The listing builds one solid part. Answer for the finished solid, in the listing's coordinates (mm). Give positions to 0.01 mm unless a question says otherwise; leave off trailing zeros. Order: outer loops, then holes, each group sorted by start corner. A loop starts at its lowest first (then second) coordinate and runs counter-clockwise, first axis right, second up. Notation, with made-up numbers: (45.25, 87.25) - (64.25, 87.25) arc R18 cw to (64.25, 116.25) - close; hole circle Ø11 at (-22, 28.5). An arc over 180 degrees is marked (long way). Answer as a JSON object with one key per item and string values. Group by question number.
Q1. The mould has two halves that part along X. Classify faces 1 (the face through (-7.535, 4.27, 0.068)), 2 (the face through (7.535, -4.27, 0.068)), 3 (the face through (-2.285, 3.584, 0.059)): released by +X, released by -X, zero draft, split by the parting line, or undercut.
Q2. A cutting plane is placed at A-A, the plane x = 0. Give the vertices of the cut face in (y, z).
Q3. A cutting plane is placed at B-B, the plane z = 2.5. Give the vertices of the cut face in (x, y), and give its area (3 significant figures).
Q4. Consider line 1 (Y direction, x = 0, z = -0.5); line 2 (X direction, y = 0.25, z = -3); line 3 (X direction, y = -3, z = -3.75). Determine where each line is inside the solid, lowest interval first.
Q5. Given pin 1 (6 mm diameter, centred on y = 5, z = -3.5, fed in from +X); pin 2 (2 mm diameter, centred on x = 7, z = -1.5, fed in from -Y); pin 3 (3 mm diameter, centred on y = 4, z = 1.5, fed in from +X), each flat-ended and moving along its own axis, determine where each tip first touches the part or whether it passes through.
from build123d import *

# Parameters (mm, degrees)
F2_SIZE  = 1.5
F4_DEPTH = 10.001


with BuildPart() as f1:
    # F0 (on Front) → F1 (revolve)
    with BuildSketch(Plane.XZ):
        Polygon((-5, 5), (-10, 5), (-10, -5), (-5, -5), (-4.25, -4.25), (-4.25, 4.25), align=None)
    revolve(axis=Axis((0, 0, 0), (0, 0, -1)))

    # F2
    f2_edges = [f1.edges().sort_by_distance(p)[0] for p in [
        (10, 0, 5),
        (10, 0, -5),
    ]]
    chamfer(f2_edges, length=F2_SIZE)

    # F3 (on face) → F4 (cut, through all)
    with BuildSketch(Plane.XY.offset(5)):
        with BuildLine():
            ThreePointArc((5, 8.660254), (0, 10), (-5, 8.660254))
            Line((-5, 8.660254), (5, 8.660254))
        make_face()
        with BuildLine():
            Line((-10, 0), (-5, 8.660254))
            ThreePointArc((-5, 8.660254), (-8.660254, 5), (-10, 0))
        make_face()
        with BuildLine():
            Line((-5, -8.660254), (-10, 0))
            ThreePointArc((-10, 0), (-8.660254, -5), (-5, -8.660254))
        make_face()
        with BuildLine():
            Line((5, -8.660254), (-5, -8.660254))
            ThreePointArc((-5, -8.660254), (0, -10), (5, -8.660254))
        make_face()
        with BuildLine():
            ThreePointArc((5, -8.660254), (8.660254, -5), (10, 0))
            Line((10, 0), (5, -8.660254))
        make_face()
        with BuildLine():
            ThreePointArc((10, 0), (8.660254, 5), (5, 8.660254))
            Line((5, 8.660254), (10, 0))
        make_face()
    extrude(amount=-F4_DEPTH, mode=Mode.SUBTRACT)


solid = f1.part
Reply:
{
 "1": {"face 1": "released by -X", "face 2": "released by +X", "face 3": "undercut"},
 "2": {"outline": "(-8.66, -4.84) - (-8.5, -5) - (-5, -5) - (-4.25, -4.25) - (-4.25, 4.25) - (-5, 5) - (-8.5, 5) - (-8.66, 4.84) - close; (4.25, -4.25) - (5, -5) - (8.5, -5) - (8.66, -4.84) - (8.66, 4.84) - (8.5, 5) - (5, 5) - (4.25, 4.25) - close"},
 "3": {"outline": "(-10, 0) - (-5, -8.66) - (5, -8.66) - (10, 0) - (5, 8.66) - (-5, 8.66) - close; hole circle Ø8.5 at (0, 0)", "area": "203 mm^2"},
 "4": {"line 1": "y = -8.66 to -4.25, 4.25 to 8.66", "line 2": "x = -9.86 to -4.24, 4.24 to 9.86", "line 3": "x = -8.27 to -3.01, 3.01 to 8.27"},
 "5": {"pin 1": "stops at x = 8.85", "pin 2": "stops at y = -6.93", "pin 3": "stops at x = 8.56"}
}
